The model under review builds one solid part; all positions refer to its coordinate system, in mm. A direction names the side the tool comes from. Round coordinates to 2 decimals unless told otherwise and drop trailing zeros. Order: outer loops, then holes, each group sorted by start corner. A loop starts at its lowest first (then second) coordinate and runs counter-clockwise, first axis right, second up.
```python
from build123d import *

# Parameters (mm, degrees)
PAD_DEPTH       = 3.7
SKETCH001_W     = 2.7
SKETCH001_H     = 1.7
POCKET_DEPTH    = 2
SKETCH002_R     = 1.3
PAD001_DEPTH    = 1
SKETCH003_W     = 1.5
SKETCH003_H     = 3.7
PAD002_DEPTH    = 0.4
POCKET001_DEPTH = 5
SKETCH005_R     = 1.3
PAD003_DEPTH    = 1
SKETCH006_W     = 1.5
SKETCH006_H     = 3.7
PAD004_DEPTH    = 0.4
POCKET002_DEPTH = 5
SKETCH008_W     = 4.7
SKETCH008_H     = 3.7
POCKET003_DEPTH = 0.4
SKETCH009_W     = 1.3
SKETCH009_H     = 3.7
POCKET004_DEPTH = 0.7
SKETCH010_W     = 2.5
SKETCH010_H     = 3.592296
POCKET005_DEPTH = 0.2
SKETCH011_W     = 2
SKETCH011_H     = 3.592296
POCKET006_DEPTH = 0.2
SKETCH012_W     = 3
SKETCH012_H     = 3.7
PAD005_DEPTH    = 1
SKETCH013_W     = 3
SKETCH013_H     = 3.7
POCKET007_DEPTH = 1
PAD006_DEPTH    = 0.4
SKETCH015_W     = 1
SKETCH015_H     = 3.7
PAD007_DEPTH    = 0.4


with BuildPart() as part:
    # Sketch → Pad (new body)
    with BuildSketch(Plane.XY):
        Polygon((0, 28), (0, 0), (4.7, 0), (4.7, 3.5), (1.3, 3.5), (1.3, 5.3), (5.8, 5.3), (5.8, 6.3), (1.3, 6.3), (1.3, 20.5), (5.8, 20.5), (5.8, 21.5), (1.3, 21.5), (1.3, 23.3), (5.8, 23.3), (5.8, 24.3), (1.3, 24.3), (1.3, 28), align=None)
    extrude(amount=PAD_DEPTH)

    # Sketch001 → Pocket (cut)
    with BuildSketch(Plane.XZ):
        with Locations((2.35, 1.85)):
            Rectangle(SKETCH001_W, SKETCH001_H)
    extrude(amount=-POCKET_DEPTH, mode=Mode.SUBTRACT)

    # Sketch002 → Pad001 (new body)
    with BuildSketch(Plane.XZ.offset(-5.3)):
        with Locations((4.4, 1.85)):
            Circle(SKETCH002_R)
    extrude(amount=PAD001_DEPTH)

    # Sketch003 → Pad002 (new body)
    with BuildSketch(Plane.XZ.offset(-5.3)):
        with Locations((5.05, 1.85)):
            Rectangle(SKETCH003_W, SKETCH003_H)
    extrude(amount=PAD002_DEPTH)

    # Sketch004 → Pocket001 (cut)
    with BuildSketch(Plane.XY.offset(3.7)):
        Polygon((5.8, 5.3), (4.3, 4.3), (5.8, 4.3), align=None)
    extrude(amount=-POCKET001_DEPTH, mode=Mode.SUBTRACT)

    # Sketch005 → Pad003 (new body)
    with BuildSketch(Plane.XZ.offset(-23.3)):
        with Locations((4.4, 1.85)):
            Circle(SKETCH005_R)
    extrude(amount=PAD003_DEPTH)

    # Sketch006 → Pad004 (new body)
    with BuildSketch(Plane.XZ.offset(-23.3)):
        with Locations((5.05, 1.85)):
            Rectangle(SKETCH006_W, SKETCH006_H)
    extrude(amount=PAD004_DEPTH)

    # Sketch007 → Pocket002 (cut)
    with BuildSketch(Plane.XY.offset(3.7)):
        Polygon((5.8, 23.3), (4.3, 22.3), (5.8, 22.3), align=None)
    extrude(amount=-POCKET002_DEPTH, mode=Mode.SUBTRACT)

    # Sketch008 → Pocket003 (cut)
    with BuildSketch(Plane.XZ):
        with Locations((2.35, 1.85)):
            Rectangle(SKETCH008_W, SKETCH008_H)
    extrude(amount=-POCKET003_DEPTH, mode=Mode.SUBTRACT)

    # Sketch009 → Pocket004 (cut)
    with BuildSketch(Plane(origin=(0, 28, 0), x_dir=(-1, 0, 0), z_dir=(0, 1, 0))):
        with Locations((-0.65, 1.85)):
            Rectangle(SKETCH009_W, SKETCH009_H)
    extrude(amount=-POCKET004_DEPTH, mode=Mode.SUBTRACT)

    # Sketch010 → Pocket005 (cut)
    with BuildSketch(Plane.XZ.offset(-4.3)):
        with Locations((4.05, 1.85)):
            Rectangle(SKETCH010_W, SKETCH010_H)
    extrude(amount=-POCKET005_DEPTH, mode=Mode.SUBTRACT)

    # Sketch011 → Pocket006 (cut)
    with BuildSketch(Plane.XZ.offset(-22.3)):
        with Locations((3.8, 1.85)):
            Rectangle(SKETCH011_W, SKETCH011_H)
    extrude(amount=-POCKET006_DEPTH, mode=Mode.SUBTRACT)

    # Sketch012 → Pad005 (new body)
    with BuildSketch(Plane.YZ.offset(1.3)):
        with Locations((25.8, 1.85)):
            Rectangle(SKETCH012_W, SKETCH012_H)
    extrude(amount=PAD005_DEPTH)

    # Sketch013 → Pocket007 (cut)
    with BuildSketch(Plane(origin=(0, 0, 0), x_dir=(0, -1, 0), z_dir=(-1, 0, 0))):
        with Locations((-25.8, 1.85)):
            Rectangle(SKETCH013_W, SKETCH013_H)
    extrude(amount=-POCKET007_DEPTH, mode=Mode.SUBTRACT)

    # Sketch014 → Pad006 (new body)
    with BuildSketch(Plane.XZ.offset(-0.4)):
        Polygon((3.7, 2.7), (3.7, 3.7), (0, 3.7), (0, 0), (3.7, 0), (3.7, 1), (1, 1), (1, 2.7), align=None)
    extrude(amount=PAD006_DEPTH)

    # Sketch015 → Pad007 (new body)
    with BuildSketch(Plane.XZ.offset(-0.4)):
        with Locations((4.2, 1.85)):
            Rectangle(SKETCH015_W, SKETCH015_H)
    extrude(amount=PAD007_DEPTH)


solid = part.part
```
(1) Consider section D-D (y = 18.75). Write out the cut boundary in (x, z).
Data:
outline: (0, 0) - (1.3, 0) - (1.3, 3.7) - (0, 3.7) - close
(2) For faces 1 (the flat face through (4, 24.3, 2)), 2 (the flat face through (4.7, 22.9, 0.3)), 3 (the flat face through (4, 20.5, 2)), 4 (the flat face through (1.3, 22, 2)), list the 3-axis set-ups (+Z, -Z, +X, -X, +Y, -Y) from which the entire face can be reached by the end or side of a thin tool; tool diameter is ignored.
Data:
face 1: +Z, -Z, +X, +Y
face 2: -Z, +X
face 3: +Z, -Z, +X
face 4: +Z, -Z
(3) Insertion check: pin 1 (1.1 mm diameter, centred on x = 3.5, z = 1, fed in from +Y); pin 2 (1 mm diameter, centred on y = 1, z = 1.5, fed in from +X); pin 3 (1.8 mm diameter, centred on y = 15, z = 2.5, fed in from +X); pin 4 (1 mm diameter, centred on x = 2, y = 18, fed in from +Z). Each pin has a flat end and moves straight along its axis. Give the tip position at first contact, or say it passes through.
Data:
pin 1: stops at y = 24.3
pin 2: stops at x = 4.7
pin 3: stops at x = 1.3
pin 4: passes through
(4) To check wall thickness, follow probe 1 along Y at (x, z) = (2.7, 2.8); probe 2 along Y at (x, z) = (1.85, 0.5); probe 3 along Y at (x, z) = (4.85, 2.35). State the ranges of each line that lie inside material, in increasing order.
Data:
probe 1: y = 0 to 3.5, 5.3 to 6.3, 20.5 to 21.5, 23.3 to 24.3
probe 2: y = 0 to 3.5, 5.3 to 6.3, 20.5 to 21.5, 23.3 to 27.3
probe 3: y = 4.67 to 6.3, 20.5 to 21.5, 22.67 to 24.3
(5) Consider section B-B (y = 1.75). Write out the cut boundary in (x, z).
Data:
outline: (0, 0) - (4.7, 0) - (4.7, 3.7) - (0, 3.7) - close; hole (1, 1) - (3.7, 1) - (3.7, 2.7) - (1, 2.7) - close
(6) Consider section A-A (x = 2.6). Write out the cut boundary in (y, z), and give its area (4 significant figures).
Data:
outline: (0, 0) - (3.5, 0) - (3.5, 3.7) - (0, 3.7) - (0, 2.7) - (2, 2.7) - (2, 1) - (0, 1) - close; (5.3, 0) - (6.3, 0) - (6.3, 3.7) - (5.3, 3.7) - close; (20.5, 0) - (21.5, 0) - (21.5, 3.7) - (20.5, 3.7) - close; (23.3, 0) - (24.3, 0) - (24.3, 3.7) - (23.3, 3.7) - close
area: 20.65 mm2
(7) Draft analysis for pull direction Y (two halves, no side actions). For faces 5 (the flat face through (1.3, 13, 2)), 6 (the flat face through (2, 0, 3)), 7 (the flat face through (2, 1, 2.7)), state which applies: pulls with the +Y half, pulls with the -Y half, needs draft (parallel to the pull), parting line crosses it, or undercut.
Data:
face 5: undercut
face 6: pulls with the -Y half
face 7: needs draft
